Model file for the job. Use its own axes, mm. Face numbers are marked on the shaded views. A direction names the side the tool comes from. Round coordinates to 2 decimals unless told otherwise and drop trailing zeros. Order: outer loops, then holes, each group sorted by start corner. A loop starts at its lowest first (then second) coordinate and runs counter-clockwise, first axis right, second up. Notation, with made-up numbers: (0, 47) - (25, 47) arc R21 ccw to (25, 55) - close; hole circle Ø7 at (65.5, 18.5). An arc over 180 degrees is marked (long way). Write item = value, one per line.
```python
from build123d import *

# Parameters (mm, degrees)
F0_W     = 4.2
F0_H     = 26.5
F0_W_2   = 23.9
F0_H_2   = 1.5
F1_DEPTH = 1
F2_DEPTH = 1.8
F3_DEPTH = 4.3
F4_W     = 17.8
F4_H     = 19.55
F4_W_2   = 30.25
F4_H_2   = 4
F4_W_3   = 42
F4_H_3   = 1
F5_DEPTH = 5.301
F7_DEPTH = 1
F8_R     = 1.5


with BuildPart() as f1:
    # F0 (on Top) → F1 (new body)
    with BuildSketch(Plane.XY):
        with Locations((18.9, -2.75)):
            Rectangle(F0_W, F0_H)
        Polygon((-16.8, -16), (16.8, -16), (16.8, 10.5), (14.3, 10.5), (14.3, 14.5), (11.95, 14.5), (-11.95, 14.5), (-14.3, 14.5), (-14.3, 10.5), (-16.8, 10.5), align=None)
        with BuildLine():
            Line((16.8, 10.5), (21, 10.5))
            Line((21, 10.5), (21, 16))
            Line((21, 16), (16.8, 16))
            Line((16.8, 16), (16.8, 14.5395311443))
            ThreePointArc((16.8, 14.5395311443), (18.2714564725, 14.7506248438), (19.075, 13.5))
            ThreePointArc((19.075, 13.5), (18.2714564725, 12.2493751562), (16.8, 12.4604688557))
            Line((16.8, 12.4604688557), (16.8, 10.5))
        make_face()
        with Locations((-18.9, -2.75)):
            Rectangle(F0_W, F0_H)
        with BuildLine():
            Line((14.3, 10.5), (16.8, 10.5))
            Line((16.8, 10.5), (16.8, 12.4604688557))
            ThreePointArc((16.8, 12.4604688557), (16.3253159421, 13.4705255898), (16.7562706956, 14.5))
            Line((16.7562706956, 14.5), (14.3, 14.5))
            Line((14.3, 14.5), (14.3, 10.5))
        make_face()
        with BuildLine():
            Line((-21, 10.5), (-16.8, 10.5))
            Line((-16.8, 10.5), (-16.8, 12.4604688557))
            ThreePointArc((-16.8, 12.4604688557), (-19.075, 13.5), (-16.8, 14.5395311443))
            Line((-16.8, 14.5395311443), (-16.8, 16))
            Line((-16.8, 16), (-21, 16))
            Line((-21, 16), (-21, 10.5))
        make_face()
        with BuildLine():
            Line((-16.8, 12.4604688557), (-16.8, 10.5))
            Line((-16.8, 10.5), (-14.3, 10.5))
            Line((-14.3, 10.5), (-14.3, 14.5))
            Line((-14.3, 14.5), (-16.7562706956, 14.5))
            ThreePointArc((-16.7562706956, 14.5), (-16.4374128162, 14.044516853), (-16.325, 13.5))
            ThreePointArc((-16.325, 13.5), (-16.4493751562, 12.9285435275), (-16.8, 12.4604688557))
        make_face()
        with BuildLine():
            Line((16.8, 14.5395311443), (16.8, 16))
            Line((16.8, 16), (11.95, 16))
            Line((11.95, 16), (11.95, 14.5))
            Line((11.95, 14.5), (14.3, 14.5))
            Line((14.3, 14.5), (16.7562706956, 14.5))
            ThreePointArc((16.7562706956, 14.5), (16.7779234767, 14.5199999437), (16.8, 14.5395311443))
        make_face()
        with Locations((0, 15.25)):
            Rectangle(F0_W_2, F0_H_2)
        with BuildLine():
            Line((-16.8, 16), (-16.8, 14.5395311443))
            ThreePointArc((-16.8, 14.5395311443), (-16.7779234767, 14.5199999437), (-16.7562706956, 14.5))
            Line((-16.7562706956, 14.5), (-14.3, 14.5))
            Line((-14.3, 14.5), (-11.95, 14.5))
            Line((-11.95, 14.5), (-11.95, 16))
            Line((-11.95, 16), (-16.8, 16))
        make_face()
    extrude(amount=F1_DEPTH)

    # F0 (on Top) → F2 (join)
    with BuildSketch(Plane.XY):
        with Locations((18.9, -2.75)):
            Rectangle(F0_W, F0_H)
        Polygon((-16.8, -16), (16.8, -16), (16.8, 10.5), (14.3, 10.5), (14.3, 14.5), (11.95, 14.5), (-11.95, 14.5), (-14.3, 14.5), (-14.3, 10.5), (-16.8, 10.5), align=None)
        with Locations((-18.9, -2.75)):
            Rectangle(F0_W, F0_H)
    extrude(amount=-F2_DEPTH)

    # F0 (on Top) → F3 (join)
    with BuildSketch(Plane.XY):
        with Locations((-18.9, -2.75)):
            Rectangle(F0_W, F0_H)
        with Locations((18.9, -2.75)):
            Rectangle(F0_W, F0_H)
    extrude(amount=-F3_DEPTH)

    # F4 (on face) → F5 (cut, through all)
    with BuildSketch(Plane.XY.offset(1)):
        Polygon((-21, 5.425), (-21, -13.925), (-0.5, -13.925), (-0.5, 5.425), (-13.3, 5.425), align=None)
        with Locations((12.1, -3.225)):
            Rectangle(F4_W, F4_H)
        with Locations((0, 14)):
            Rectangle(F4_W_2, F4_H_2)
        Polygon((-13.3, 5.425), (-0.5, 5.425), (1.7, 5.425), (1.7, 10.425), (-13.3, 10.425), align=None)
        with Locations((0, -15.5)):
            Rectangle(F4_W_3, F4_H_3)
    extrude(amount=-F5_DEPTH, mode=Mode.SUBTRACT)

    # F6 (on face) → F7 (cut)
    with BuildSketch(Plane(origin=(0, 0, -1.8), x_dir=(1, 0, 0), z_dir=(0, 0, -1))):
        Polygon((-13.3, -5.425), (-14.3, -5.425), (-14.3, -10.5), (-14.3, -12), (14.3, -12), (14.3, -10.5), (14.3, -6.55), (3.2, -6.55), (3.2, -5.425), (1.7, -5.425), (1.7, -10.425), (-13.3, -10.425), align=None)
    extrude(amount=-F7_DEPTH, mode=Mode.SUBTRACT)

    # F8
    f8_edges = [f1.edges().sort_by_distance(p)[0] for p in [
        (-21, 16, 0.5),
        (21, 16, 0.5),
        (21, 10.5, -2.15),
        (-21, 10.5, -2.15),
        (-21, 5.425, -1.65),
        (21, 6.55, -1.65),
        (-15.125, 16, 0.5),
        (15.125, 16, 0.5),
        (15.125, 12, 0.5),
        (-15.125, 12, 0.5),
        (3.2, 6.55, 0.1),
        (3.2, -13, -0.4),
        (-0.5, -13.925, -0.4),
        (-13.3, 10.425, 0.1),
        (1.7, 5.425, 0.1),
    ]]
    fillet(f8_edges, radius=F8_R)


solid = f1.part
```
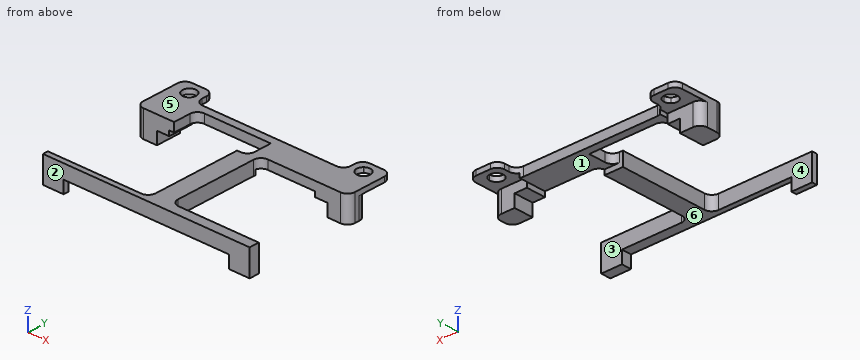
1) Cut at C-C (x = 11.5). Write the cut outline in (y, z), and give its area (3 significant figures).
Conclusion:
outline = (-15, -1.8) - (-13, -1.8) - (-13, 1) - (-15, 1) - close; (6.55, -0.8) - (12, -0.8) - (12, 1) - (6.55, 1) - close
area = 15.4 mm^2
2) 3-axis set-ups, long thin cutter, end or side, ignore diameter. For the marked faces 4, 5 and 6: which of +Z, -Z, +X, -X, +Y, -Y reach the whole face in a straight line?
Conclusion:
face_4 = +Z, -Z, -X
face_5 = +Z, +X, -X, +Y, -Y
face_6 = -Z, +Y, -Y
3) Cut at A-A (z = -2.6). Write the cut outline in (x, y) (3 decimals), and give its area (3 significant figures).
Conclusion:
outline = (-21, -15) - (-16.8, -15) - (-16.8, -13.925) - (-21, -13.925) - close; (-21, 6.925) arc R1.5 ccw to (-19.5, 5.425) - (-16.8, 5.425) - (-16.8, 10.5) - (-19.5, 10.5) arc R1.5 ccw to (-21, 9) - close; (16.8, -15) - (21, -15) - (21, -13) - (16.8, -13) - close; (16.8, 6.55) - (19.5, 6.55) arc R1.5 ccw to (21, 8.05) - (21, 9) arc R1.5 ccw to (19.5, 10.5) - (16.8, 10.5) - close
area = 48.9 mm^2
4) Wall check: line 1 along Y through (x, z) = (-17.7, 0.2) (3 decimals); line 2 along X through (y, z) = (13.5, 0.8) (3 decimals); line 3 along Y through (x, z) = (11.5, 0.5). Give the ranges that are in metal, low to high.
Conclusion:
line_1 = -15 to -13.925, 5.425 to 12.125, 14.875 to 16
line_2 = -21 to -19.075, -16.325 to -15.125, 15.125 to 16.325, 19.075 to 21
line_3 = -15 to -13, 6.55 to 12
5) Flat gauge pins, fed straight in: pin 1 Ø0.6 at (y, z) = (11, -0.5) entering from +X; pin 2 Ø1.5 at (y, z) = (5.5, -3) entering from +X; pin 3 Ø1.5 at (x, y) = (5, -2.5) entering from -Z; pin 4 Ø1.6 at (x, z) = (10.5, -1) entering from +Y. Where does each tip first touch, or does it go through?
Conclusion:
pin_1 = 14.3
pin_2 = -16.8
pin_3 = through
pin_4 = 12
6) Mould opens along Y. For the marked faces 1, 2 and 3 say: +Y half, -Y half, draft (parallel to the pull), parting line (faces both ways), or undercut.
Conclusion:
face_1 = draft
face_2 = -Y half
face_3 = undercut
7) Cut at B-B (x = -17.7). Write the cut outline in (y, z) (3 decimals), and give its area (3 significant figures).
Conclusion:
outline = (-15, -4.3) - (-13.925, -4.3) - (-13.925, 1) - (-15, 1) - close; (5.425, -4.3) - (10.5, -4.3) - (10.5, 0) - (12.125, 0) - (12.125, 1) - (5.425, 1) - close; (14.875, 0) - (16, 0) - (16, 1) - (14.875, 1) - close
area = 35.3 mm^2
8) Cut at D-D (y = -4.5). Write the cut outline in (x, z).
Conclusion:
outline = (-0.5, -1.8) - (3.2, -1.8) - (3.2, 1) - (-0.5, 1) - close
